```python
from build123d import *

# Parameters (mm, degrees)
F0_R     = 10.9982
F1_DEPTH = 7.000011


with BuildPart() as f1:
    # F0 (on Top) → F1 (new body)
    with BuildSketch(Plane.XY):
        with BuildLine():
            ThreePointArc((2.088246, -6.887012), (10.590885, -2.184077), (13.97, 6.92603))
            ThreePointArc((13.97, 6.92603), (13.967218, 7.204808), (13.958874, 7.483476))
            ThreePointArc((13.958874, 7.483476), (13.090268, 11.805146), (10.918322, 15.641025))
            ThreePointArc((10.918322, 15.641025), (2.319695, 20.702093), (-7.462199, 18.736046))
            ThreePointArc((-7.462199, 18.736046), (-10.770573, 15.822976), (-13.006568, 12.024077))
            ThreePointArc((-13.006568, 12.024077), (-13.090268, 2.046913), (-6.496674, -5.441432))
            ThreePointArc((-6.496674, -5.441432), (-2.319695, -6.850033), (2.088246, -6.887012))
        make_face()
        with Locations((0, 6.92603)):
            Circle(F0_R, mode=Mode.SUBTRACT)
        with BuildLine():
            ThreePointArc((13.958874, 7.483476), (13.967218, 7.204808), (13.97, 6.92603))
            ThreePointArc((13.97, 6.92603), (10.590885, -2.184077), (2.088246, -6.887012))
            ThreePointArc((2.088246, -6.887012), (10.903349, -8.961172), (19.09199, -12.828255))
            ThreePointArc((19.09199, -12.828255), (21.183867, -4.773264), (27.485263, 0.662841))
            ThreePointArc((27.485263, 0.662841), (20.291579, 3.219431), (13.958874, 7.483476))
        make_face()
        with BuildLine():
            ThreePointArc((-7.462199, 18.736046), (2.319695, 20.702093), (10.918322, 15.641025))
            ThreePointArc((10.918322, 15.641025), (8.307046, 24.312208), (7.561717, 33.337321))
            ThreePointArc((7.561717, 33.337321), (-0.460048, 31.121444), (-8.318551, 33.86056))
            ThreePointArc((-8.318551, 33.86056), (-6.935781, 26.352352), (-7.462199, 18.736046))
        make_face()
        with BuildLine():
            ThreePointArc((47.015656, -12.152889), (40.70993, -0.473), (27.485263, 0.662841))
            ThreePointArc((27.485263, 0.662841), (21.183867, -4.773264), (19.09199, -12.828255))
            ThreePointArc((19.09199, -12.828255), (19.843858, -15.396303), (20.367595, -18.020398))
            ThreePointArc((20.367595, -18.020398), (32.416208, -26.108701), (45.144031, -19.137889))
            ThreePointArc((45.144031, -19.137889), (46.53964, -15.768591), (47.015656, -12.152889))
        make_face()
        with Locations((33.045656, -12.152889)):
            Circle(F0_R, mode=Mode.SUBTRACT)
        with BuildLine():
            ThreePointArc((-19.166712, -13.745312), (-13.355798, -8.793694), (-6.496674, -5.441432))
            ThreePointArc((-6.496674, -5.441432), (-13.090268, 2.046913), (-13.006568, 12.024077))
            ThreePointArc((-13.006568, 12.024077), (-19.210395, 5.427054), (-26.653708, 0.269023))
            ThreePointArc((-26.653708, 0.269023), (-21.119709, -4.877403), (-19.075656, -12.152889))
            ThreePointArc((-19.075656, -12.152889), (-19.098439, -12.950401), (-19.166712, -13.745312))
        make_face()
        with BuildLine():
            ThreePointArc((20.367595, -18.020398), (19.843858, -15.396303), (19.09199, -12.828255))
            ThreePointArc((19.09199, -12.828255), (19.479087, -15.48592), (20.367595, -18.020398))
        make_face()
        with BuildLine():
            ThreePointArc((11.420443, 37.038098), (9.409778, 35.272481), (7.561717, 33.337321))
            ThreePointArc((7.561717, 33.337321), (9.669774, 35.001389), (11.420443, 37.038098))
        make_face()
        with BuildLine():
            ThreePointArc((-8.318551, 33.86056), (-0.460048, 31.121444), (7.561717, 33.337321))
            ThreePointArc((7.561717, 33.337321), (9.409778, 35.272481), (11.420443, 37.038098))
            ThreePointArc((11.420443, 37.038098), (13.317366, 40.863836), (13.97, 45.083867))
            ThreePointArc((13.97, 45.083867), (9.878282, 54.962148), (0, 59.053867))
            ThreePointArc((0, 59.053867), (-13.265566, 49.46401), (-8.318551, 33.86056))
        make_face()
        with Locations((0, 45.083867)):
            Circle(F0_R, mode=Mode.SUBTRACT)
        with BuildLine():
            ThreePointArc((-45.144031, -19.137889), (-30.206188, -25.831277), (-19.166712, -13.745312))
            ThreePointArc((-19.166712, -13.745312), (-19.098439, -12.950401), (-19.075656, -12.152889))
            ThreePointArc((-19.075656, -12.152889), (-21.119709, -4.877403), (-26.653708, 0.269023))
            ThreePointArc((-26.653708, 0.269023), (-29.253636, 0.901911), (-31.788038, 1.760389))
            ThreePointArc((-31.788038, 1.760389), (-44.81702, -4.629864), (-45.144031, -19.137889))
        make_face()
        with Locations((-33.045656, -12.152889)):
            Circle(F0_R, mode=Mode.SUBTRACT)
        with BuildLine():
            ThreePointArc((45.144031, -19.137889), (32.416208, -26.108701), (20.367595, -18.020398))
            ThreePointArc((20.367595, -18.020398), (20.047579, -29.054393), (15.81854, -39.250799))
            ThreePointArc((15.81854, -39.250799), (33.010768, -32.882439), (45.144031, -19.137889))
        make_face()
        with BuildLine():
            ThreePointArc((13.97, 45.083867), (13.317366, 40.863836), (11.420443, 37.038098))
            ThreePointArc((11.420443, 37.038098), (21.136171, 42.277954), (32.081037, 43.713701))
            ThreePointArc((32.081037, 43.713701), (17.969761, 55.418428), (0, 59.053867))
            ThreePointArc((0, 59.053867), (9.878282, 54.962148), (13.97, 45.083867))
        make_face()
        with BuildLine():
            ThreePointArc((-31.788038, 1.760389), (-29.253636, 0.901911), (-26.653708, 0.269023))
            ThreePointArc((-26.653708, 0.269023), (-29.148861, 1.262621), (-31.788038, 1.760389))
        make_face()
        with BuildLine():
            ThreePointArc((-47.899577, 16.315187), (-50.980529, -1.7579), (-45.144031, -19.137889))
            ThreePointArc((-45.144031, -19.137889), (-44.81702, -4.629864), (-31.788038, 1.760389))
            ThreePointArc((-31.788038, 1.760389), (-41.18375, 7.554529), (-47.899577, 16.315187))
        make_face()
    extrude(amount=-F1_DEPTH)


solid = f1.part
```
Geometry check sheet. Reference: the model listing, model coordinates, mm. A direction names the side the tool comes from. Give positions to 0.01 mm unless a question says otherwise; leave off trailing zeros. Loops run counter-clockwise (first coordinate to the right, second up) from the corner with the lowest first, then second, coordinate; pieces in that order, holes last. Notation, with made-up numbers: M 19,20.5 L 77,20.5 A16 cw 77,43.5 Z; hole C -34,-23.5 d5. An arc over 180 degrees is marked long. Write item = value, one per line. Start each with the question number.
1. Tool access check on faces 4 (the face through (-29.11, 1.25, -3.45)), 5 (the face through (-13.445, -8.853, -3.451)), 6 (the face through (19.47, -15.45, -3.45)). Record the directions out of +Z, -Z, +X, -X, +Y, -Y that give a thin tool (end or side, any length) a straight path to the whole face; none if there is none.
2. Go/stop test with flat-tipped pins: P1, Ø4, axis at x = -2, y = -9.5, coming from the -Z side; P2, Ø10, axis at x = -14.5, y = 13.5, coming from the -Z side; P3, Ø4, axis at y = 36, z = -3, coming from the -X side; P4, Ø1.5, axis at x = -21, z = -4.5, coming from the -Y side. Record where each tip stops, or that it passes through.
3. Draft check along X on faces 1 (the face through (8.33, 24.19, -3.45)), 2 (the face through (-13.187, 49.696, -3.451)), 3 (the face through (20.39, 3.17, -3.45)). Enter one of: +X half, -X half, draft (parallel to the pull), parting line (faces both ways), or undercut.
4. Thickness scan on probe 1 along X at (y, z) = (15.5, -3.5); probe 2 along X at (y, z) = (4.5, -0.75); probe 3 along X at (y, z) = (17, -3.5). Record the ranges inside material, lowest first.
5. Section check C-C, the plane y = 46.5. Enter the section's corners in (x, z), plus the area to 3 significant figures.
6. Section check A-A, the plane x = -4.5. Enter the section's corners in (y, z), plus the area to 3 significant figures.
7. Section check B-B, the plane x = -24.5. Enter the section's corners in (y, z).
8. Section check D-D, the plane z = -3.25. Enter the section's corners in (x, y) (1 decimal).
Values follow:
q1.face_4 = +Z, -Z, +Y
q1.face_5 = +Z, -Z, -Y
q1.face_6 = +Z, -Z
q2.P1 = through
q2.P2 = -7
q2.P3 = -12.04
q2.P4 = -20.37
q3.face_1 = +X half
q3.face_2 = -X half
q3.face_3 = undercut
q4.probe_1 = -48.25 to -47.47, -11.03 to -6.89, 6.89 to 11.03
q4.probe_2 = -50.94 to -37.18, -20.32 to -10.73, 10.73 to 18
q4.probe_3 = -9.68 to -4.41, 4.41 to 10.37
q5.outline = M -13.9,-7 L -10.91,-7 L -10.91,0 L -13.9,0 Z; M 10.91,-7 L 29.83,-7 L 29.83,0 L 10.91,0 Z
q5.area = 153 mm^2
q6.outline = M -6.3,-7 L -3.11,-7 L -3.11,0 L -6.3,0 Z; M 16.96,-7 L 35.05,-7 L 35.05,0 L 16.96,0 Z; M 55.12,-7 L 58.31,-7 L 58.31,0 L 55.12,0 Z
q6.area = 171 mm^2
q7.outline = M -23.2,-7 L -19.08,-7 L -19.08,0 L -23.2,0 Z; M -5.23,-7 L 1.53,-7 L 1.53,0 L -5.23,0 Z
q8.outline = M -47.9,16.3 A37.6 ccw -45.1,-19.1 A14 ccw -19.2,-13.7 A30.5 cw -6.5,-5.4 A14 ccw 2.1,-6.9 A43.2 cw 19.1,-12.8 A14 ccw 20.4,-18 A30.5 cw 15.8,-39.3 A37.6 ccw 45.1,-19.1 A14 ccw 47,-12.2 A14 ccw 27.5,0.7 A30.5 cw 14,7.5 A14 ccw 10.9,15.6 A43.2 cw 7.6,33.3 A14 ccw 11.4,37 A30.5 cw 32.1,43.7 A37.6 ccw 0,59.1 A14 ccw -8.3,33.9 A30.5 cw -7.5,18.7 A14 ccw -13,12 A43.2 cw -26.7,0.3 A14 ccw -31.8,1.8 A30.5 cw Z; hole C -33,-12.2 d22; hole C 0,6.9 d22; hole C 0,45.1 d22; hole C 33,-12.2 d22
